Work out the finished part from the listing and answer in its coordinate system (mm). Face numbers are marked on the shaded views. A direction names the side the tool comes from. Coordinates: 2 decimals unless noted, no trailing zeros. Order: outer loops, then holes, each group sorted by start corner. A loop starts at its lowest first (then second) coordinate and runs counter-clockwise, first axis right, second up.
1. Flat-ended cylindrical pins translate along their axes: pin 1 Ø1 at (x, z) = (0, -1.5) entering from +Y; pin 2 Ø1.3 at (x, y) = (5, 0) entering from +Z; pin 3 Ø1 at (x, z) = (2.5, -1) entering from -Y. Find the tip coordinate at first contact, or state that the pin passes through.
2. The part is cut by section D-D, the plane x = 1.25. Give the vertices of the cut face in (y, z).
3. A tool of negligible diameter and unlimited length cuts with its end or side. For the marked faces 4, 5 and 6, from which of +Z, -Z, +X, -X, +Y, -Y can it reach the whole face along a straight path? Write none if from no direction.
4. Determine the mould class of the marked faces 1, 2 and 3 for opening direction X: +X half, -X half, draft (parallel to the pull), parting line (faces both ways), or undercut.
5. Find the intervals of material crossed by probe 1 along X at (y, z) = (-0.3, -0.5); probe 2 along X at (y, z) = (-0.25, 5.75); probe 3 along Y at (x, z) = (5.5, 7.5), in increasing order.
6. The part is cut by section C-C, the plane y = 0.7. Give the vertices of the cut face in (x, z), then the cut area to 3 significant figures.
7. The part is cut by section B-B, the plane z = 4.25. Give the vertices of the cut face in (x, y), then the cut area to 3 significant figures.
8. The part is cut by section A-A, the plane z = -0.75. Give the vertices of the cut face in (x, y), then the cut area to 3 significant figures.
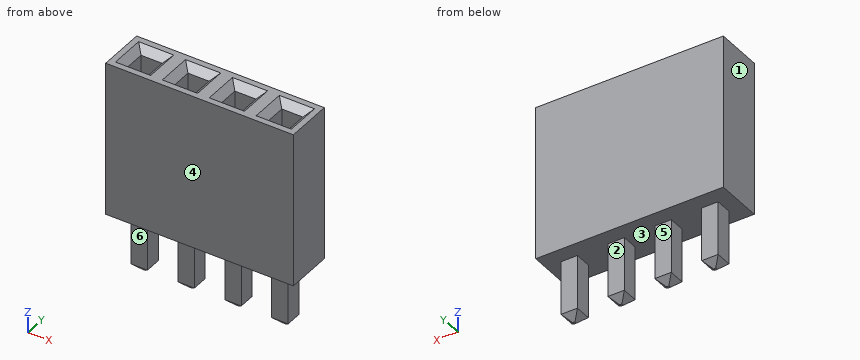
Autodesk Inventor part; units mm, degrees
ref_plane "YZ Plane" through (0, 0, 0) normal (1, 0, 0) x (0, 1, 0)
ref_plane "XZ Plane" through (0, 0, 0) normal (0, 1, 0) x (-1, 0, 0)
ref_plane "XY Plane" through (0, 0, 0) normal (0, 0, 1) x (1, 0, 0)
sketch "Sketch1" plane through (0, 0, 0) normal (0, 0, 1) x (1, 0, 0)
  line L0 (1.27, -1.27) -> (-1.27, -1.27)
  line L1 (-1.27, -1.27) -> (-1.27, 1.27)
  line L2 (-1.27, 1.27) -> (1.27, 1.27)
  line L3 (1.27, 1.27) -> (1.27, -1.27)
  line L4 (1.27, -1.27) -> (-1.27, 1.27) construction
  line L5 (-1.27, -1.27) -> (1.27, 1.27) construction
  point P0 (0, 0)
  dimension "d0" = 2.54
  dimension "d1" = 2.54
extrude "Extrusion1" add sketch "Sketch1" along normal blind 8.382
sketch "Sketch2" plane through (0, 0, 8.382) normal (0, 0, 1) x (1, 0, 0)
  line L0 (0.5715, 0.5715) -> (-0.5715, 0.5715)
  line L1 (-0.5715, 0.5715) -> (-0.5715, -0.5715)
  line L2 (-0.5715, -0.5715) -> (0.5715, -0.5715)
  line L3 (0.5715, -0.5715) -> (0.5715, 0.5715)
  line L4 (0.5715, 0.5715) -> (-0.5715, -0.5715) construction
  line L5 (-0.5715, 0.5715) -> (0.5715, -0.5715) construction
  point P0 (0, 0)
  dimension "d4" = 1.143
extrude "Extrusion2" cut sketch "Sketch2" against normal blind 6.35
chamfer "Chamfer1" distance 0.381 angle 45 4 edges at (0, 0.5715, 8.382) (-0.5715, 0, 8.382) (0, -0.5715, 8.382) (0.5715, 0, 8.382)
sketch "Sketch3" plane through (0, 0, 0) normal (0, 0, -1) x (-1, 0, 0)
  line L0 (0.4445, -0.4445) -> (-0.4445, -0.4445)
  line L1 (-0.4445, -0.4445) -> (-0.4445, 0.4445)
  line L2 (-0.4445, 0.4445) -> (0.4445, 0.4445)
  line L3 (0.4445, 0.4445) -> (0.4445, -0.4445)
  line L4 (0.4445, -0.4445) -> (-0.4445, 0.4445) construction
  line L5 (-0.4445, -0.4445) -> (0.4445, 0.4445) construction
  point P0 (0, 0)
  dimension "d10" = 0.889
extrude "Extrusion3" add sketch "Sketch3" along normal blind 3.302
chamfer "Chamfer2" distance 0.381 angle 45 4 edges at (0, 0.4445, -3.302) (-0.4445, 0, -3.302) (0, -0.4445, -3.302) (0.4445, 0, -3.302)
pattern_linear "Rectangular Pattern1" count 4 spacing 2.54 along (1, 0, 0) of "Extrusion1", "Extrusion2", "Chamfer1", "Extrusion3", "Chamfer2"
equation "\"d1\" = d0"
properties part number "4  female pin"
Geometry says:
1. pin 1: stops at y = 0.44
1. pin 2: stops at z = 8.16
1. pin 3: stops at y = -0.44
2. outline: (-1.27, 0) - (1.27, 0) - (1.27, 8.38) - (-1.27, 8.38) - close
3. face 4: +Z, -Z, +X, -X, -Y
3. face 5: -Z, +X, -X, +Y
3. face 6: -Z, +X, -X, -Y
4. face 1: -X half
4. face 2: draft
4. face 3: undercut
5. probe 1: x = -0.44 to 0.44, 2.1 to 2.98, 4.64 to 5.52, 7.18 to 8.06
5. probe 2: x = -1.27 to -0.57, 0.57 to 1.97, 3.11 to 4.51, 5.65 to 7.05, 8.19 to 8.89
5. probe 3: y = -1.27 to -0.57, 0.57 to 1.27
6. outline: (-1.27, 0) - (8.89, 0) - (8.89, 8.38) - (8.57, 8.38) - (8.32, 8.13) - (6.92, 8.13) - (6.67, 8.38) - (6.03, 8.38) - (5.78, 8.13) - (4.38, 8.13) - (4.13, 8.38) - (3.49, 8.38) - (3.24, 8.13) - (1.84, 8.13) - (1.59, 8.38) - (0.95, 8.38) - (0.7, 8.13) - (-0.7, 8.13) - (-0.95, 8.38) - (-1.27, 8.38) - close
6. area: 83.5 mm2
7. outline: (-1.27, -1.27) - (8.89, -1.27) - (8.89, 1.27) - (-1.27, 1.27) - close; hole (-0.57, -0.57) - (0.57, -0.57) - (0.57, 0.57) - (-0.57, 0.57) - close; hole (1.97, -0.57) - (3.11, -0.57) - (3.11, 0.57) - (1.97, 0.57) - close; hole (4.51, -0.57) - (5.65, -0.57) - (5.65, 0.57) - (4.51, 0.57) - close; hole (7.05, -0.57) - (8.19, -0.57) - (8.19, 0.57) - (7.05, 0.57) - close
7. area: 20.6 mm2
8. outline: (-0.44, -0.44) - (0.44, -0.44) - (0.44, 0.44) - (-0.44, 0.44) - close; (2.1, -0.44) - (2.98, -0.44) - (2.98, 0.44) - (2.1, 0.44) - close; (4.64, -0.44) - (5.52, -0.44) - (5.52, 0.44) - (4.64, 0.44) - close; (7.18, -0.44) - (8.06, -0.44) - (8.06, 0.44) - (7.18, 0.44) - close
8. area: 3.16 mm2
